from build123d import *

# Parameters (mm, degrees)
F0_R     = 14
F1_DEPTH = 300
F2_W     = 39.96696
F2_H     = 44.953362
F2_R     = 14
F3_DEPTH = 25


with BuildPart() as f1:
    # F0 (on Top) → F1 (new body)
    with BuildSketch(Plane.XY):
        Circle(F0_R)
    extrude(amount=F1_DEPTH)

    # F2 (on face) → F3 (join)
    with BuildSketch(Plane.XY.offset(300)):
        Rectangle(F2_W, F2_H)
        Circle(F2_R, mode=Mode.SUBTRACT)
    extrude(amount=-F3_DEPTH)


solid = f1.part
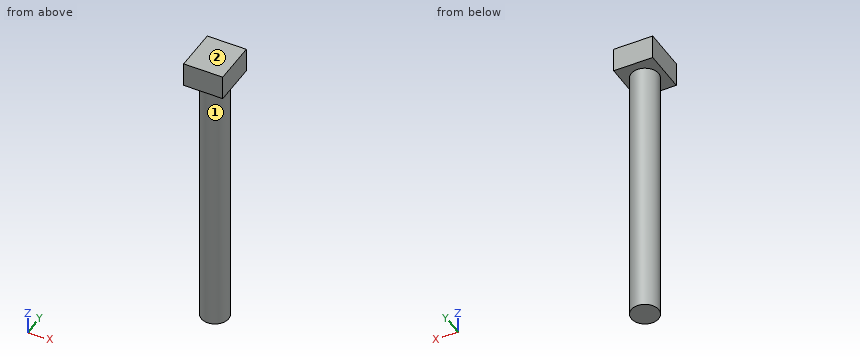
Geometry check sheet. Reference: the model listing, model coordinates, mm. Face numbers are marked on the shaded views. A direction names the side the tool comes from. Round coordinates to 2 decimals unless told otherwise and drop trailing zeros. Write each loop counter-clockwise with the first axis right and the second up, starting at its lowest first coordinate (ties: lowest second). Pieces come first, ordered by that corner, then holes.
Item 1: Material ranges on line 1 along Z through (x, y) = (-12.5, 18.5); line 2 along X through (y, z) = (-0.5, 200); line 3 along Y through (x, z) = (0, 62.5), recorded low to high.
Determined:
line 1: z = 275 to 300
line 2: x = -13.99 to 13.99
line 3: y = -14 to 14
Item 2: Go/stop test with flat-tipped pins: pin 1 Ø2 at (x, z) = (-11.5, 34.5) entering from +Y; pin 2 Ø2 at (x, y) = (-14.5, 13) entering from -Z; pin 3 Ø1 at (x, z) = (-0.5, 119) entering from -Y. Record where each tip stops, or that it passes through.
Determined:
pin 1: stops at y = 9.26
pin 2: stops at z = 275
pin 3: stops at y = -14
Item 3: Section check A-A (x = 0). Record the boundary of the cut face in (y, z).
Determined:
outline: (-22.48, 275) - (-14, 275) - (-14, 0) - (14, 0) - (14, 275) - (22.48, 275) - (22.48, 300) - (-22.48, 300) - close
Item 4: Section check C-C (y = -18). Record the boundary of the cut face in (x, z), plus the area to 3 significant figures.
Determined:
outline: (-19.98, 275) - (19.98, 275) - (19.98, 300) - (-19.98, 300) - close
area: 999 mm2
Item 5: Section check B-B (y = 0). Record the boundary of the cut face in (x, z).
Determined:
outline: (-19.98, 275) - (-14, 275) - (-14, 0) - (14, 0) - (14, 275) - (19.98, 275) - (19.98, 300) - (-19.98, 300) - close
Item 6: Access from +Z, -Z, +X, -X, +Y, -Y to the whole of each face (thin tool, end or side, straight path). Record for the marked faces 1 and 2.
Determined:
face 1: -Z
face 2: +Z, +X, -X, +Y, -Y
